Check sheet for the modelled part. Datum: model origin and axes. Units: mm. Round coordinates to 2 decimals unless told otherwise and drop trailing zeros. Write each loop counter-clockwise with the first axis right and the second up, starting at its lowest first coordinate (ties: lowest second). Pieces come first, ordered by that corner, then holes. Notation, with made-up numbers: (22, 25) -> (49, 25) arc R8 cw to (49, 30) -> close; hole circle Ø2 at (26.5, 10). An arc over 180 degrees is marked (long way). One line per item, written item: value.
from build123d import *

# Parameters (mm, degrees)
F0_R     = 22
F1_DEPTH = 3
F2_DEPTH = 3
F4_DEPTH = 25


with BuildPart() as f1:
    # F0 (on Front) → F1 (new body)
    with BuildSketch(Plane.XZ):
        Polygon((0, 101.624342229), (-23.4537052032, 87.530419444), (-50.8121711145, 88.0092620132), (-64.0767142408, 64.0767142408), (-88.0092620132, 50.8121711145), (-87.530419444, 23.4537052032), (-101.624342229, 0), (-87.530419444, -23.4537052032), (-88.0092620132, -50.8121711145), (-64.0767142408, -64.0767142409), (-50.8121711145, -88.0092620132), (-23.4537052032, -87.530419444), (0, -101.624342229), (23.4537052032, -87.530419444), (50.8121711145, -88.0092620132), (64.0767142409, -64.0767142408), (88.0092620132, -50.8121711145), (87.530419444, -23.4537052032), (101.624342229, 0), (87.530419444, 23.4537052032), (88.0092620132, 50.8121711145), (64.0767142408, 64.0767142408), (50.8121711145, 88.0092620132), (23.4537052032, 87.530419444), align=None)
        Circle(F0_R, mode=Mode.SUBTRACT)
    extrude(amount=F1_DEPTH)

    # F0 (on Front) → F2 (join)
    with BuildSketch(Plane.XZ):
        Polygon((0, 101.624342229), (-23.4537052032, 87.530419444), (-50.8121711145, 88.0092620132), (-64.0767142408, 64.0767142408), (-88.0092620132, 50.8121711145), (-87.530419444, 23.4537052032), (-101.624342229, 0), (-87.530419444, -23.4537052032), (-88.0092620132, -50.8121711145), (-64.0767142408, -64.0767142409), (-50.8121711145, -88.0092620132), (-23.4537052032, -87.530419444), (0, -101.624342229), (23.4537052032, -87.530419444), (50.8121711145, -88.0092620132), (64.0767142409, -64.0767142408), (88.0092620132, -50.8121711145), (87.530419444, -23.4537052032), (101.624342229, 0), (87.530419444, 23.4537052032), (88.0092620132, 50.8121711145), (64.0767142408, 64.0767142408), (50.8121711145, 88.0092620132), (23.4537052032, 87.530419444), align=None)
        Circle(F0_R, mode=Mode.SUBTRACT)
    extrude(amount=F2_DEPTH)

    # F3 (on face) → F4 (cut)
    with BuildSketch(Plane.XZ.offset(3)):
        Polygon((-85.7229544101, -1.5), (-85.7229544101, 1.5), (-100.7229544101, 1.5), (-100.7229544101, 14.0027841553), (-117.494545877, 14.0027841553), (-117.494545877, -1.5), (-100.7229544101, -1.5), align=None)
    extrude(amount=-F4_DEPTH, mode=Mode.SUBTRACT)


solid = f1.part
Item 1: Mould release check, pull along Z, two halves, no side actions. Record for faces 1 (the flat face through (-11.89, -1.48, -94.48)), 2 (the cylindrical face through (-4.769, -1.479, -21.477)), 3 (the flat face through (76.21, -1.48, 57.35)): pulls with the +Z half, pulls with the -Z half, needs draft (parallel to the pull), parting line crosses it, or undercut.
Answer:
face 1: pulls with the -Z half
face 2: undercut
face 3: pulls with the +Z half
Item 2: Depth check by flat-ended pin: P1, Ø1.5, axis at x = -15.5, z = -77, coming from the +Y side. Enter the tip coordinate at first touch or a pass-through.
Answer:
P1: stops at y = 0
Item 3: Sectioned sample at D-D on x = 48. Enter the section's corners in (y, z), and give its area (3 significant figures).
Answer:
outline: (-3, -87.96) -> (0, -87.96) -> (0, 87.96) -> (-3, 87.96) -> close
area: 528 mm^2
Item 4: Sectioned sample at B-B on x = 6. Enter the section's corners in (y, z), and give its area (3 significant figures).
Answer:
outline: (-3, -98.02) -> (0, -98.02) -> (0, -21.17) -> (-3, -21.17) -> close; (-3, 21.17) -> (0, 21.17) -> (0, 98.02) -> (-3, 98.02) -> close
area: 461 mm^2
Item 5: Sectioned sample at C-C on z = 61. Enter the section's corners in (x, y).
Answer:
outline: (-69.63, -3) -> (69.63, -3) -> (69.63, 0) -> (-69.63, 0) -> close
Item 6: Sectioned sample at A-A on y = -0.6. Enter the section's corners in (x, z), and give its area (3 significant figures).
Answer:
outline: (-100.72, -1.5) -> (-87.53, -23.45) -> (-88.01, -50.81) -> (-64.08, -64.08) -> (-50.81, -88.01) -> (-23.45, -87.53) -> (0, -101.62) -> (23.45, -87.53) -> (50.81, -88.01) -> (64.08, -64.08) -> (88.01, -50.81) -> (87.53, -23.45) -> (101.62, 0) -> (87.53, 23.45) -> (88.01, 50.81) -> (64.08, 64.08) -> (50.81, 88.01) -> (23.45, 87.53) -> (0, 101.62) -> (-23.45, 87.53) -> (-50.81, 88.01) -> (-64.08, 64.08) -> (-88.01, 50.81) -> (-87.53, 23.45) -> (-100.72, 1.5) -> (-85.72, 1.5) -> (-85.72, -1.5) -> close; hole circle Ø44 at (0, 0)
area: 27,000 mm^2
Item 7: Thickness scan on line 1 (Z direction, x = 0, y = -1.1); line 2 (X direction, y = -2.5, z = -0.5); line 3 (Z direction, x = 3, y = -0.9). Record the ranges inside material, lowest first.
Answer:
line 1: z = -101.62 to -22, 22 to 101.62
line 2: x = -85.72 to -21.99, 21.99 to 101.32
line 3: z = -99.82 to -21.79, 21.79 to 99.82
